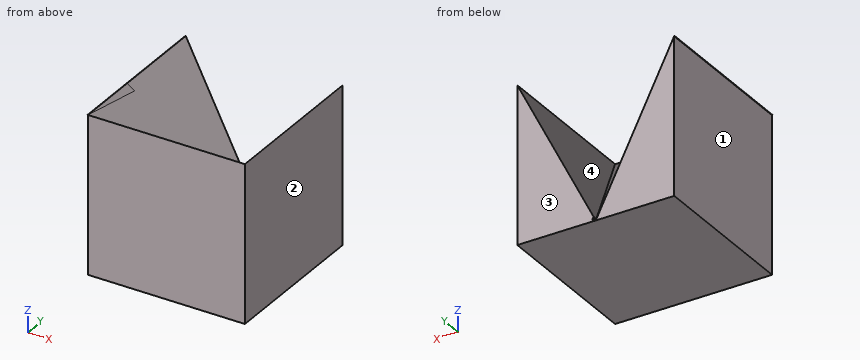
```python
from build123d import *

# Parameters (mm, degrees)
SKETCH1_W           = 40
SKETCH1_H           = 40
BOSS_EXTRUDE1_DEPTH = 40
CUT_EXTRUDE1_DEPTH  = 40
CUT_EXTRUDE3_DEPTH  = 40
CUT_EXTRUDE5_DEPTH  = 1
BOSS_EXTRUDE2_DEPTH = 26
CUT_EXTRUDE7_DEPTH  = 5
CUT_EXTRUDE8_DEPTH  = 5
CUT_EXTRUDE9_DEPTH  = 5
SKETCH10_W          = 40
SKETCH10_H          = 40
CUT_EXTRUDE10_DEPTH = 50
SKETCH11_W          = 56.739460666
SKETCH11_H          = 49.026259181
CUT_EXTRUDE11_DEPTH = 50


with BuildPart() as part:
    # Sketch1 → Boss-Extrude1 (new body)
    with BuildSketch(Plane.XY):
        with Locations((20, 20)):
            Rectangle(SKETCH1_W, SKETCH1_H)
    extrude(amount=BOSS_EXTRUDE1_DEPTH)

    # Sketch2 → Cut-Extrude1 (cut)
    with BuildSketch(Plane(origin=(0, 20, 20), x_dir=(1, 0, 0), z_dir=(0, 0.707106781, 0.707106781))):
        Polygon((40, -28.284271247), (0, -28.284271247), (20, 28.284271247), align=None)
    extrude(amount=CUT_EXTRUDE1_DEPTH, mode=Mode.SUBTRACT)

    # Sketch4 → Cut-Extrude3 (cut)
    with BuildSketch(Plane(origin=(16, 0, -8), x_dir=(0.447213595, 0, 0.894427191), z_dir=(-0.894427191, 0, 0.447213595))):
        Polygon((8.94427191, 40), (53.66563146, 40), (53.66563146, 0), align=None)
    extrude(amount=CUT_EXTRUDE3_DEPTH, mode=Mode.SUBTRACT)

    # Sketch5 → Cut-Extrude5 (cut)
    with BuildSketch(Plane(origin=(16, 0, 8), x_dir=(-0.447213595, 0, 0.894427191), z_dir=(-0.894427191, 0, -0.447213595))):
        Polygon((35.77708764, 0), (-8.94427191, 40), (29.348133104, 45.420073385), align=None)
    extrude(amount=-CUT_EXTRUDE5_DEPTH, mode=Mode.SUBTRACT)

    # Sketch6 → Boss-Extrude2 (add)
    with BuildSketch(Plane(origin=(16, 0, 8), x_dir=(-0.447213595, 0, 0.894427191), z_dir=(-0.894427191, 0, -0.447213595))):
        Polygon((35.77708764, 40), (35.77708764, 0), (-8.94427191, 40), align=None)
    extrude(amount=BOSS_EXTRUDE2_DEPTH)

    # Sketch7 → Cut-Extrude7 (cut)
    with BuildSketch(Plane(origin=(16, 0, 8), x_dir=(0.447213595, 0, -0.894427191), z_dir=(0.894427191, 0, 0.447213595))):
        Polygon((2.978893099, 34.664402987), (-35.77708764, 31.206354084), (-35.77708764, 16), (-33.326207642, 17.315280227), (-35.77708764, 0), align=None)
    extrude(amount=CUT_EXTRUDE7_DEPTH, mode=Mode.SUBTRACT)

    # Sketch8 → Cut-Extrude8 (cut)
    with BuildSketch(Plane(origin=(-15.685739325, 4.964580059, 31.37147865), x_dir=(-0.896620465, -0.069212396, -0.437357275), z_dir=(0.442799889, -0.140147395, -0.885599778))):
        Polygon((-21.749837593, 8.458308195), (-18.716733371, 11.192845531), (-17.494290991, -6.252250535), align=None)
    extrude(amount=-CUT_EXTRUDE8_DEPTH, mode=Mode.SUBTRACT)

    # Sketch9 → Cut-Extrude9 (cut)
    with BuildSketch(Plane(origin=(15.970902322, -3.85667421, 8.59577521), x_dir=(-0.450614766, 0.108815038, 0.88606186), z_dir=(-0.86130493, 0.207989032, -0.463567018))):
        Polygon((35.4424744, 15.010038766), (34.947973708, 15.305740233), (35.4424744, 0), align=None)
    extrude(amount=-CUT_EXTRUDE9_DEPTH, mode=Mode.SUBTRACT)

    # Sketch10 → Cut-Extrude10 (cut)
    with BuildSketch(Plane(origin=(0, 0, 0), x_dir=(-1, 0, 0), z_dir=(0, 0, -1))):
        with Locations((-20, 20)):
            Rectangle(SKETCH10_W, SKETCH10_H)
    extrude(amount=CUT_EXTRUDE10_DEPTH, mode=Mode.SUBTRACT)

    # Sketch11 → Cut-Extrude11 (cut)
    with BuildSketch(Plane.ZY):
        with Locations((11.546622416, 24.513129591)):
            Rectangle(SKETCH11_W, SKETCH11_H)
    extrude(amount=CUT_EXTRUDE11_DEPTH, mode=Mode.SUBTRACT)


solid = part.part
```
Source: CAD feature listing. Evaluate the final solid. Frame: model axes, mm. Face numbers are marked on the shaded views. Coordinates: 2 decimals unless noted, no trailing zeros. Loops run counter-clockwise (first coordinate to the right, second up) from the corner with the lowest first, then second, coordinate; pieces in that order, holes last. Notation, with made-up numbers: (0, 32) -> (15, 32) arc R24 cw to (15, 70) -> close; hole circle Ø10 at (33, 52.25). An arc over 180 degrees is marked (long way). One line per item, written item: value. Start each with the question number.
Q1. Contact query for flat-ended pins moving along their axis: P1, Ø20, axis at y = 18.5, z = 10.5, coming from the -X side; P2, Ø10, axis at x = 21, y = 11, coming from the +Z side. Output: stop coordinate, or through.
Q2. Line query: line 1 along X through (y, z) = (35, 24); line 2 along X through (y, z) = (16.5, 13.5); line 3 along X through (y, z) = (35.5, 10). Output: solid intervals per line, ascending.
Q3. Section query C-C, the plane x = 16. Return the cut outline in (y, z).
Q4. Mould query, pull axis X, two halves, no side actions, for the marked faces 1, 2, 3 and 4. Classes: pulls with the +X half, pulls with the -X half, needs draft (parallel to the pull), parting line crosses it, or undercut.
Q5. Section query A-A, the plane z = 21. Return the cut outline in (x, y), and give its area (3 significant figures).
Q6. Section query B-B, the plane y = 29.5. Return the cut outline in (x, z), and give its area (3 significant figures).
Q7. Section query D-D, the plane y = 3. Return the cut outline in (x, z).
Results:
1. P1: x = 0
1. P2: z = 34
2. line 1: 0 to 8, 32 to 40
2. line 2: 0 to 40
2. line 3: 0 to 15, 25 to 40
3. outline: (0, 0) -> (40, 0) -> (40, 8) -> (32, 8) -> (0, 40) -> close
4. face 1: pulls with the -X half
4. face 2: pulls with the +X half
4. face 3: needs draft
4. face 4: undercut
5. outline: (0, 0) -> (40, 0) -> (40, 40) -> (30.5, 40) -> (30.5, 19) -> (9.5, 19) -> (9.5, 40) -> (0, 40) -> close
5. area: 1,160 mm^2
6. outline: (-0.17, 39.92) -> (0, 39.92) -> (0, 0) -> (40, 0) -> (40, 40) -> (25.25, 10.5) -> (14.75, 10.5) -> (0, 40) -> close
6. area: 855 mm^2
7. outline: (-0.17, 39.92) -> (0, 39.92) -> (0, 0) -> (40, 0) -> (40, 40) -> (38.5, 37) -> (1.5, 37) -> (0, 40) -> close
